```python
from build123d import *

# Parameters (mm, degrees)
SKETCH2_R          = 2.10058
CUT_EXTRUDE1_DEPTH = 38


with BuildPart() as part:
    # Sketch1 → Revolve1 (revolve)
    with BuildSketch(Plane.XY):
        Polygon((0, 0), (0, 37), (19.5, 37), (20, 36.5), (20, 25.5), (19.5, 25), (12, 25), (12, 0.5), (11.5, 0), align=None)
    revolve(axis=Axis((0, 0, 0), (0, 1, 0)))

    # Sketch2 → Cut-Extrude1 (cut, through all)
    with BuildSketch(Plane(origin=(0, 37, 0), x_dir=(1, 0, 0), z_dir=(0, 1, 0))):
        with Locations((0, 15.5)):
            Circle(SKETCH2_R)
        with Locations((13.423393759, -7.75)):
            Circle(SKETCH2_R)
        with Locations((-13.423393759, -7.75)):
            Circle(SKETCH2_R)
    extrude(amount=-CUT_EXTRUDE1_DEPTH, mode=Mode.SUBTRACT)


solid = part.part
```
Geometry: final body of the model. Coordinates: model frame, mm. A direction names the side the tool comes from. Round coordinates to 2 decimals unless told otherwise and drop trailing zeros. Order: outer loops, then holes, each group sorted by start corner. A loop starts at its lowest first (then second) coordinate and runs counter-clockwise, first axis right, second up. Notation, with made-up numbers: (-12, 14) -> (-2, 14) arc R22 cw to (-2, 37) -> close; hole circle Ø9 at (69, -12). An arc over 180 degrees is marked (long way). Use one line per item in the form item = value.
(1) Draft query along Z for faces 1 (the face through (8.4, 25, -8.9)), 2 (the face through (12.97, 31.08, 9.8)), 3 (the face through (-11.48, 31.08, 8.55)), 4 (the face through (-4.336, 30.923, 19.524)). Return one class per face: pulls with the +Z half, pulls with the -Z half, needs draft (parallel to the pull), parting line crosses it, or undercut.
Results list:
face_1 = needs draft
face_2 = undercut
face_3 = undercut
face_4 = parting line crosses it
(2) Section A-A on z = 0. Return loops of the section in (x, y).
Results list:
outline = (-20, 25.5) -> (-19.5, 25) -> (-12, 25) -> (-12, 0.5) -> (-11.5, 0) -> (11.5, 0) -> (12, 0.5) -> (12, 25) -> (19.5, 25) -> (20, 25.5) -> (20, 36.5) -> (19.5, 37) -> (-19.5, 37) -> (-20, 36.5) -> close
(3) First-contact query: pin 1 Ø1.5 at (x, y) = (4, 31.5) entering from +Z; pin 2 Ø3 at (x, y) = (-6, 8) entering from -Z; pin 3 Ø5.5 at (x, z) = (0, -15.5) entering from -Y. Flat tips, straight axial feed; report the tip coordinate or a pass-through.
Results list:
pin_1 = 19.73
pin_2 = -11.12
pin_3 = 25
(4) Section D-D on z = 7.75. Count the separate pieces of the cut face and the enclosed holes in it, and give its area (3 significant figures).
Results list:
separate_pieces = 3
enclosed_holes = 0
area = 799 mm^2
(5) Section B-B on y = 3. Return loops of the section in (x, z).
Results list:
outline = circle Ø24 at (0, 0)
(6) Section C-C on y = 28. Return loops of the section in (x, z), and give its area (3 significant figures).
Results list:
outline = circle Ø40 at (0, 0); hole circle Ø4.2 at (-13.42, 7.75); hole circle Ø4.2 at (0, -15.5); hole circle Ø4.2 at (13.42, 7.75)
area = 1,220 mm^2
(7) Access query for faces 5 (the face through (0, 0, 0)), 6 (the face through (-11.99, 12.58, -0.53)). Directions: +Z, -Z, +X, -X, +Y, -Y. A direction counts if a zero-diameter tool reaches every point of the face in a straight line with its end or side. Return the directions, or none.
Results list:
face_5 = +Z, -Z, +X, -X, -Y
face_6 = -Y
(8) Ray query, probe 1 along X at (y, z) = (29, 7) (3 decimals); probe 2 along Y at (x, z) = (12, 1); probe 3 along Z at (x, y) = (12, 25.5). Return the intervals inside material, ascending. Write a range as [from, to].
Results list:
probe_1 = [-18.735, -15.386], [-11.461, 11.461], [15.386, 18.735]
probe_2 = [25, 37]
probe_3 = [-16, 6.21], [9.29, 16]
